Autodesk Inventor part; units mm, degrees
ref_plane "YZ Plane" through (0, 0, 0) normal (1, 0, 0) x (0, 1, 0)
ref_plane "XZ Plane" through (0, 0, 0) normal (0, 1, 0) x (-1, 0, 0)
ref_plane "XY Plane" through (0, 0, 0) normal (0, 0, 1) x (1, 0, 0)
sketch "Sketch1" plane through (0, 0, 0) normal (0, 0, 1) x (1, 0, 0)
  circle A0 centre (0, 0) radius 1.5
  dimension "d0" = 3
extrude "Extrusion1" add sketch "Sketch1" along normal blind 4.49
fillet "Fillet1" radius 1.5 1 edges at (-1.5, 0, 4.49)
sketch "Sketch2" plane through (0, 0, 0) normal (0, 0, -1) x (-1, 0, 0)
  circle A0 centre (0, 0) radius 1.5
  circle A1 centre (0, 0) radius 1.875
  dimension "d4" = 3.75
extrude "Extrusion2" add sketch "Sketch2" along normal blind 1 contours A0 | A1
sketch "Sketch3" plane through (0, 0, -1) normal (0, 0, -1) x (-1, 0, 0)
  circle A0 centre (0, 0) radius 1.875
  line L0 (-1.52, 0.25) -> (-1.02, 0.25)
  line L1 (-1.02, 0.25) -> (-1.02, -0.25)
  line L2 (-1.02, -0.25) -> (-1.52, -0.25)
  line L3 (-1.52, -0.25) -> (-1.52, 0.25)
  line L4 (1.02, 0.25) -> (1.52, 0.25)
  line L5 (1.52, 0.25) -> (1.52, -0.25)
  line L6 (1.52, -0.25) -> (1.02, -0.25)
  line L7 (1.02, -0.25) -> (1.02, 0.25)
  dimension "d7" = 0.5
  dimension "d8" = 0.5
  dimension "d9" = 0.5
  dimension "d10" = 0.5
  dimension "d11" = 0.25
  dimension "d12" = 0.25
  dimension "d13" = 1.02
  dimension "d14" = 1.02
sketch "Sketch4" plane through (0, 0, 0) normal (1, 0, 0) x (0, 1, 0)
  line L0 (0, -0.5) -> (0, -3.75)
  line L1 (-2, -5.75) -> (-4, -5.75)
  line L2 (-1.875, -1) -> (1.875, -1)
  arc A0 (-2, -5.75) -> (0, -3.75) centre (-2, -3.75) ccw
  line L3 (1.875, 0) -> (-1.875, 0)
  point P0 (0, 0)
  point P1 (0, -5.75)
  dimension "d16" = 4
  dimension "d17" = 5.25
  dimension "d18" = 2
  dimension "d19" = 1.875
  dimension "d21" = 0.5
sweep "Sweep1" add profiles "Sketch3" path "Sketch4" path curves L0 A0 L1 contours L0 L1 L2 L3 | L4 L5 L6 L7
properties part number "led"
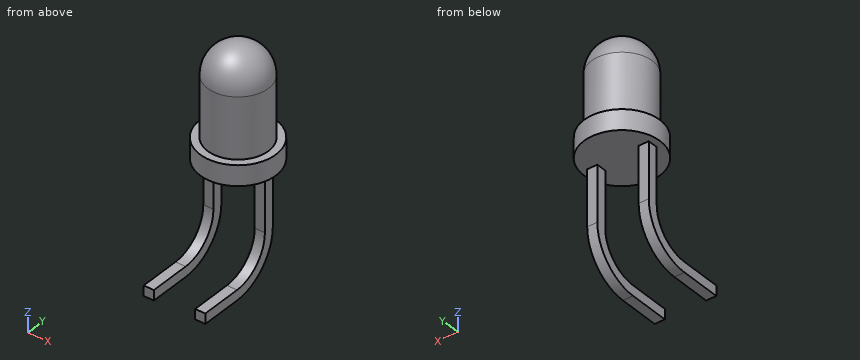
Work out the finished part from the listing and answer in its coordinate system (mm). Give positions to 0.01 mm unless a question says otherwise; leave off trailing zeros. Loops run counter-clockwise (first coordinate to the right, second up) from the corner with the lowest first, then second, coordinate; pieces in that order, holes last. Notation, with made-up numbers: (70.25, 30) - (105.25, 30) arc R20 cw to (105.25, 64) - close; hole circle Ø4 at (-39.5, -37.5). An arc over 180 degrees is marked (long way). Answer in a Markdown table with one row per item. Add a question column.
Q1. Each of these flat-tipped pins is pushed along its axis until it touches: P1, Ø1.9, axis at x = -0.5, y = 0.5, coming from the -Z side; P2, Ø0.6, axis at x = 1.5, z = -2.5, coming from the +Y side; P3, Ø1, axis at y = 1, z = 0, coming from the +X side. Where does it stop, or does it pass through?
Q2. The part is cut by section D-D (z = 2.5). Determine the outline of the cut face in (x, y).
Q3. Consider line 1 along Z through (x, y) = (1.1, -2.15); line 2 along Z through (x, y) = (1.3, -0.95); line 3 along Y through (x, z) = (1.25, -2.25). Determine where each line is inside the solid, lowest interval first.
Q4. The part is cut by section C-C (x = 0). Determine the outline of the cut face in (y, z) (3 decimals), and give its area (3 significant figures).
Q5. The part is cut by section A-A (z = -3.5). Determine the outline of the cut face in (x, y), and give its area (3 significant figures).
Q6. The part is cut by section B-B (y = -0.6). Determine the outline of the cut face in (x, z), and give its area (3 significant figures).
Solution:
| question | item | result |
|---|---|---|
| 1 | P1 | stops at z = -5.22 |
| 1 | P2 | stops at y = 0.25 |
| 1 | P3 | stops at x = 1.81 |
| 2 | outline | circle Ø3 at (0, 0) |
| 3 | line 1 | z = -6 to -5.5 |
| 3 | line 2 | z = -5.74 to -5.15, -1 to 0 |
| 3 | line 3 | y = -0.25 to 0.25 |
| 4 | outline | (-1.875, -1) - (1.875, -1) - (1.875, 0) - (1.5, 0) - (1.5, 2.99) arc R1.5 ccw to (-1.5, 2.99) - (-1.5, 0) - (-1.875, 0) - close |
| 4 | area | 16.3 mm² |
| 5 | outline | (-1.52, -0.25) - (-1.02, -0.25) - (-1.02, 0.25) - (-1.52, 0.25) - close; (1.02, -0.25) - (1.52, -0.25) - (1.52, 0.25) - (1.02, 0.25) - close |
| 5 | area | 0.500 mm² |
| 6 | outline | (-1.78, -1) - (1.78, -1) - (1.78, 0) - (1.37, 0) - (1.37, 2.99) arc R1.37 ccw to (-1.37, 2.99) - (-1.37, 0) - (-1.78, 0) - close; (-1.52, -5.51) - (-1.02, -5.51) - (-1.02, -4.8) - (-1.52, -4.8) - close; (1.02, -5.51) - (1.52, -5.51) - (1.52, -4.8) - (1.02, -4.8) - close |
| 6 | area | 15.5 mm² |
